```python
from build123d import *

# Parameters (mm, degrees)
SKETCH1_W           = 62
SKETCH1_H           = 36.5
BOSS_EXTRUDE1_DEPTH = 12.7
SKETCH2_R           = 1.905
CUT_EXTRUDE1_DEPTH  = 12.7


with BuildPart() as part:
    # Sketch1 → Boss-Extrude1 (new body)
    with BuildSketch(Plane(origin=(0, 0, 0), x_dir=(1, 0, 0), z_dir=(0, 1, 0))):
        Rectangle(SKETCH1_W, SKETCH1_H)
    extrude(amount=BOSS_EXTRUDE1_DEPTH)

    # Sketch2 → Cut-Extrude1 (cut)
    with BuildSketch(Plane(origin=(0, 12.7, 0), x_dir=(1, 0, 0), z_dir=(0, 1, 0))):
        with Locations((26.555, 13.805)):
            Circle(SKETCH2_R)
        with Locations((26.555, -13.805)):
            Circle(SKETCH2_R)
        with Locations((-26.555, 13.805)):
            Circle(SKETCH2_R)
        with Locations((-26.555, -13.805)):
            Circle(SKETCH2_R)
    extrude(amount=-CUT_EXTRUDE1_DEPTH, mode=Mode.SUBTRACT)


solid = part.part
```
Input: part model. Units: mm. Frame: model coordinates. Round coordinates to 2 decimals unless told otherwise and drop trailing zeros. Write each loop counter-clockwise with the first axis right and the second up, starting at its lowest first coordinate (ties: lowest second). Pieces come first, ordered by that corner, then holes. Notation, with made-up numbers: (57, 9.5) - (90, 9.5) arc R11 cw to (90, 18.5) - close; hole circle Ø10 at (61.25, 37.25). An arc over 180 degrees is marked (long way). Write item = value, one per line.
(1) Section query B-B on y = 9.5. Output: boundary loops of the cut face in (x, z) (3 decimals).
Geometry check:
outline = (-31, -18.25) - (31, -18.25) - (31, 18.25) - (-31, 18.25) - close; hole circle Ø3.81 at (-26.555, -13.805); hole circle Ø3.81 at (-26.555, 13.805); hole circle Ø3.81 at (26.555, -13.805); hole circle Ø3.81 at (26.555, 13.805)
(2) Pull-direction query (Z, two-part tool) for faces 1 (the flat face through (0, 6, 18.25)), 2 (the flat face through (0, 6, -18.25)), 3 (the cylindrical face through (-24.795, 6.439, 14.535)), 4 (the flat face through (31, 6, 0)); classes: +Z half, -Z half, draft (parallel to the pull), parting line (faces both ways), or undercut.
Geometry check:
face_1 = +Z half
face_2 = -Z half
face_3 = undercut
face_4 = draft
(3) Material intervals for probe 1 along X at (y, z) = (4.75, -14); probe 2 along X at (y, z) = (4.25, 15); probe 3 along Z at (x, y) = (-27, 1.25), sorted ascending.
Geometry check:
probe_1 = -31 to -28.45, -24.66 to 24.66, 28.45 to 31
probe_2 = -31 to -28.04, -25.07 to 25.07, 28.04 to 31
probe_3 = -18.25 to -15.66, -11.95 to 11.95, 15.66 to 18.25
(4) Section query A-A on z = -15. Output: boundary loops of the cut face in (x, y).
Geometry check:
outline = (-31, 0) - (-28.04, 0) - (-28.04, 12.7) - (-31, 12.7) - close; (-25.07, 0) - (25.07, 0) - (25.07, 12.7) - (-25.07, 12.7) - close; (28.04, 0) - (31, 0) - (31, 12.7) - (28.04, 12.7) - close
